The listing builds one solid part. Answer for the finished solid, in the listing's coordinates (mm). A direction names the side the tool comes from. Coordinates: 2 decimals unless noted, no trailing zeros. Write each loop counter-clockwise with the first axis right and the second up, starting at its lowest first coordinate (ties: lowest second). Pieces come first, ordered by that corner, then holes.
from build123d import *

# Parameters (mm, degrees)
F1_DEPTH = 6.35
F3_DEPTH = 9.525
F4_R     = 5.08


with BuildPart() as f1:
    # F0 (on Front) → F1 (new body)
    with BuildSketch(Plane.XZ):
        Polygon((0, 63.5), (0, 0), (-57.15, 0), (-57.15, -60.325), (60.325, -60.325), (60.325, 63.5), align=None)
    extrude(amount=F1_DEPTH)

    # F2 (on face) → F3 (join)
    with BuildSketch(Plane.XZ.offset(6.35)):
        Polygon((-57.15, -53.975), (-57.15, -60.325), (60.325, -60.325), (60.325, 63.5), (53.975, 63.5), (53.975, -53.975), align=None)
    extrude(amount=F3_DEPTH)

    # F4
    f4_edges = [f1.edges().sort_by_distance(p)[0] for p in [
        (60.325, -7.9375, -60.325),
    ]]
    fillet(f4_edges, radius=F4_R)


solid = f1.part
Q1. Which of the six approach directions +Z, -Z, +X, -X, +Y, -Y give full straight-line access (tool end or side, diameter ignored) to faces 1 (the face through (0, -3, 32)), 2 (the face through (-57.15, -4, -30)), 3 (the face through (10, -6.35, -7))?
Answers below:
face 1: +Z, -X, +Y, -Y
face 2: +Z, -Z, -X, +Y, -Y
face 3: +Z, -X, -Y
Q2. Given pin 1 (6 mm diameter, centred on x = 21, y = -13.5, fed in from +Z) (3 decimals); pin 2 (3 mm diameter, centred on x = -23, y = -2.5, fed in from +Z); pin 3 (4 mm diameter, centred on y = -9.5, z = 18, fed in from -X) (3 decimals), each flat-ended and moving along its own axis, determine where each tip first touches the part or whether it passes through.
Answers below:
pin 1: stops at z = -53.975
pin 2: stops at z = 0
pin 3: stops at x = 53.975
Q3. The part is cut by section C-C, the plane z = 35. Write down the section's boundary in (x, y) (3 decimals), then the cut area to 3 significant figures.
Answers below:
outline: (0, -6.35) - (53.975, -6.35) - (53.975, -15.875) - (60.325, -15.875) - (60.325, 0) - (0, 0) - close
area: 444 mm2
Q4. Find the intervals of material crossed by probe 1 along Y at (x, z) = (44, 12.5); probe 2 along Z at (x, y) = (42, -14.5) (3 decimals); probe 3 along X at (y, z) = (-14, 41) (3 decimals), in increasing order.
Answers below:
probe 1: y = -6.35 to 0
probe 2: z = -60.325 to -53.975
probe 3: x = 53.975 to 60.325
Q5. The part is cut by section B-B, the plane x = 11.5. Write down the section's boundary in (y, z) (3 decimals).
Answers below:
outline: (-15.875, -60.325) - (0, -60.325) - (0, 63.5) - (-6.35, 63.5) - (-6.35, -53.975) - (-15.875, -53.975) - close
Q6. The part is cut by section D-D, the plane y = -13.75. Write down the section's boundary in (x, z) (3 decimals), then the cut area to 3 significant figures.
Answers below:
outline: (-57.15, -60.325) - (55.245, -60.325) arc R5.08 ccw to (60.325, -55.245) - (60.325, 63.5) - (53.975, 63.5) - (53.975, -53.975) - (-57.15, -53.975) - close
area: 1,490 mm2
Q7. The part is cut by section A-A, the plane y = -4.75. Write down the section's boundary in (x, z) (3 decimals), then the cut area to 3 significant figures.
Answers below:
outline: (-57.15, -60.325) - (55.245, -60.325) arc R5.08 ccw to (60.325, -55.245) - (60.325, 63.5) - (0, 63.5) - (0, 0) - (-57.15, 0) - close
area: 10,900 mm2
